from build123d import *

# Parameters (mm, degrees)
SKETCH1_R               = 7
BOSS_EXTRUDE1_DEPTH     = 13
SKETCH2_W               = 56.2
SKETCH2_H               = 16
CUT_EXTRUDE1_DEPTH      = 10
CUT_EXTRUDE2_REACH      = 56.246
SKETCH3_W               = 15
SKETCH3_H               = 16
SKETCH4_W               = 15
SKETCH4_H               = 23
BOSS_EXTRUDE2_DEPTH     = 16
SKETCH5_W               = 13
SKETCH5_H               = 21
CUT_EXTRUDE3_DEPTH      = 12
CUT_EXTRUDE4_REACH      = 59.303
SKETCH6_R               = 1.5
SKETCH6_R_2             = 1.05
SKETCH7_R               = 2.5
SKETCH7_R_2             = 1.5
BOSS_EXTRUDE3_DEPTH     = 10
CHAMFER1_SIZE           = 7
CHAMFER1_SIZE2          = 0.612420645
CUT_EXTRUDE5_REACH      = 103.55
CUT_EXTRUDE5_END_RADIUS = 7
SKETCH8_R               = 1.25
CUT_EXTRUDE6_REACH      = 103.55
CUT_EXTRUDE6_END_RADIUS = 7
SKETCH9_R               = 1.25


with BuildPart() as part:
    # Sketch1 → Boss-Extrude1 (new body)
    with BuildSketch(Plane(origin=(0, 0, 0), x_dir=(1, 0, 0), z_dir=(0, 1, 0))):
        Polygon((-28.1, -7), (-28.1, 10), (-48.1, 10), (-48.1, -23), (-28.1, -23), (28.1, -23), (48.1, -23), (48.1, 10), (28.1, 10), (28.1, -7), align=None)
        with Locations(Location((-38.1, 0, 0), (0, 0, 90))):
            Circle(SKETCH1_R, mode=Mode.SUBTRACT)
        with Locations(Location((38.1, 0, 0), (0, 0, 90))):
            Circle(SKETCH1_R, mode=Mode.SUBTRACT)
    extrude(amount=BOSS_EXTRUDE1_DEPTH)

    # Sketch2 → Cut-Extrude1 (cut)
    with BuildSketch(Plane(origin=(0, 13, 0), x_dir=(1, 0, 0), z_dir=(0, 1, 0))):
        with Locations((0, -15)):
            Rectangle(SKETCH2_W, SKETCH2_H)
    extrude(amount=-CUT_EXTRUDE1_DEPTH, mode=Mode.SUBTRACT)

    # Sketch3 → Cut-Extrude2 (cut, up to next)
    with BuildSketch(Plane(origin=(0, 3, 0), x_dir=(1, 0, 0), z_dir=(0, 1, 0)), mode=Mode.PRIVATE) as cut_extrude2_sk1:
        with Locations((0, -15)):
            Rectangle(SKETCH3_W, SKETCH3_H)
    cut_extrude2_tool1 = extrude(cut_extrude2_sk1.sketch, amount=-CUT_EXTRUDE2_REACH, mode=Mode.PRIVATE) & part.part
    add(cut_extrude2_tool1.solids().sort_by_distance((0, 3, 15))[0], mode=Mode.SUBTRACT)


with BuildPart() as cut_extrude2_piece_1:
    # of the separate pieces the step leaves, piece 1, a body of its own (cut_extrude2_pieces)
    add(part.part.solids().sort_by_distance((28.1, 0, 7))[0])



with BuildPart() as cut_extrude2_piece_2:
    # of the separate pieces the step leaves, piece 2, a body of its own (cut_extrude2_pieces)
    add(part.part.solids().sort_by_distance((-28.1, 0, 7))[0])


with BuildPart() as cut_extrude2_piece_1_1:
    add(cut_extrude2_piece_1.part)

    add(cut_extrude2_piece_2.part)  # Boss-Extrude2 merges Cut-Extrude2 piece 2
    # Sketch4 → Boss-Extrude2 (add)
    with BuildSketch(Plane.XY.offset(23)):
        with Locations((0, 11.5)):
            Rectangle(SKETCH4_W, SKETCH4_H)
    extrude(amount=-BOSS_EXTRUDE2_DEPTH)

    # Sketch5 → Cut-Extrude3 (cut)
    with BuildSketch(Plane.XY.offset(23)):
        with Locations((0, 11.5)):
            Rectangle(SKETCH5_W, SKETCH5_H)
    extrude(amount=-CUT_EXTRUDE3_DEPTH, mode=Mode.SUBTRACT)

    # Sketch6 → Cut-Extrude4 (cut, up to next)
    with BuildSketch(Plane.XY.offset(11), mode=Mode.PRIVATE) as cut_extrude4_sk1:
        with Locations((0, 11.464154045)):
            Circle(SKETCH6_R)
    cut_extrude4_tool1 = extrude(cut_extrude4_sk1.sketch, amount=-CUT_EXTRUDE4_REACH, mode=Mode.PRIVATE) & cut_extrude2_piece_1_1.part
    # Sketch6 → Cut-Extrude4 (cut, up to next)
    with BuildSketch(Plane.XY.offset(11), mode=Mode.PRIVATE) as cut_extrude4_sk2:
        with Locations((0, 6.964154045)):
            Circle(SKETCH6_R_2)
    cut_extrude4_tool2 = extrude(cut_extrude4_sk2.sketch, amount=-CUT_EXTRUDE4_REACH, mode=Mode.PRIVATE) & cut_extrude2_piece_1_1.part
    add(cut_extrude4_tool1.solids().sort_by_distance((0, 11.464154, 11))[0], mode=Mode.SUBTRACT)
    add(cut_extrude4_tool2.solids().sort_by_distance((0, 6.964154, 11))[0], mode=Mode.SUBTRACT)

    # Sketch7 → Boss-Extrude3 (add)
    with BuildSketch(Plane(origin=(0, 0, 7), x_dir=(-1, 0, 0), z_dir=(0, 0, -1))):
        with Locations(Location((0, 11.464154045, 0), (0, 0, 180))):
            Circle(SKETCH7_R)
        with Locations(Location((0, 11.464154045, 0), (0, 0, 180))):
            Circle(SKETCH7_R_2, mode=Mode.SUBTRACT)
    extrude(amount=BOSS_EXTRUDE3_DEPTH)

    # Chamfer1
    chamfer1_edges = [cut_extrude2_piece_1_1.edges().sort_by_distance(p)[0] for p in [
        (-2.5, 11.464154045, -3),
    ]]
    chamfer1_side = [cut_extrude2_piece_1_1.faces().sort_by_distance(p)[0] for p in [
        (-2.5, 11.464154045, 2),
    ]]
    chamfer(chamfer1_edges, length=CHAMFER1_SIZE, length2=CHAMFER1_SIZE2, reference=chamfer1_side[0])

    # Cut-Extrude5: up to this cylinder (the profile starts outside it)
    cut_extrude5_end = Plane(origin=(-38.1, 6.5, 0), z_dir=(0, -1, 0)) * Cylinder(CUT_EXTRUDE5_END_RADIUS, 222.1, mode=Mode.PRIVATE)
    # Sketch8 → Cut-Extrude5 (cut, up to the surface)
    with BuildSketch(Plane.ZY.offset(48.1), mode=Mode.PRIVATE) as cut_extrude5_sk1:
        with Locations((0, 6.5)):
            Circle(SKETCH8_R)
    cut_extrude5_tool1 = extrude(cut_extrude5_sk1.sketch, amount=-CUT_EXTRUDE5_REACH, mode=Mode.PRIVATE) - cut_extrude5_end
    add(cut_extrude5_tool1.solids().sort_by_distance((-48.1, 6.5, 0))[0], mode=Mode.SUBTRACT)

    # Cut-Extrude6: up to this cylinder (the profile starts outside it)
    cut_extrude6_end = Plane(origin=(38.1, 6.5, 0), z_dir=(0, -1, 0)) * Cylinder(CUT_EXTRUDE6_END_RADIUS, 222.1, mode=Mode.PRIVATE)
    # Sketch9 → Cut-Extrude6 (cut, up to the surface)
    with BuildSketch(Plane(origin=(48.1, 0, 0), x_dir=(0, 0, -1), z_dir=(1, 0, 0)), mode=Mode.PRIVATE) as cut_extrude6_sk1:
        with Locations(Location((0, 6.5, 0), (0, 0, 180))):
            Circle(SKETCH9_R)
    cut_extrude6_tool1 = extrude(cut_extrude6_sk1.sketch, amount=-CUT_EXTRUDE6_REACH, mode=Mode.PRIVATE) - cut_extrude6_end
    add(cut_extrude6_tool1.solids().sort_by_distance((48.1, 6.5, 0))[0], mode=Mode.SUBTRACT)


solid = cut_extrude2_piece_1_1.part
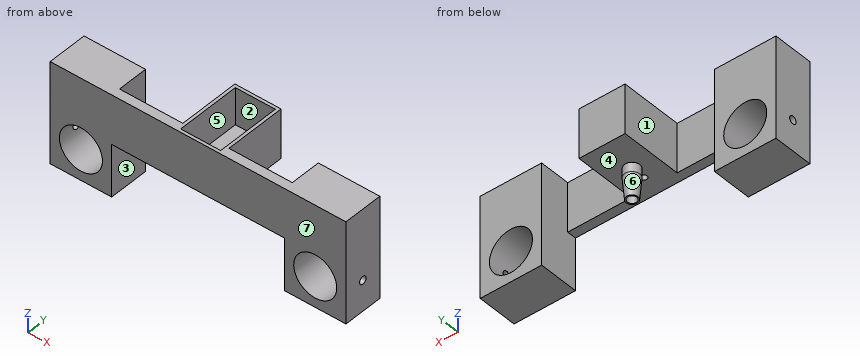
Input: part model. Units: mm. Frame: model coordinates. Face numbers are marked on the shaded views. A direction names the side the tool comes from. Give positions to 0.01 mm unless a question says otherwise; leave off trailing zeros. Write each loop counter-clockwise with the first axis right and the second up, starting at its lowest first coordinate (ties: lowest second). Pieces come first, ordered by that corner, then holes. Notation, with made-up numbers: M 0,17.5 L 15,17.5 A20 cw 15,49.5 Z; hole C 54.25,35.5 d7. An arc over 180 degrees is marked long. Write item = value, one per line. Start each with the question number.
1) Draft query along Y for the marked faces 4, 5, 6 and 7. Return one class per face: +Y half, -Y half, draft (parallel to the pull), parting line (faces both ways), or undercut.
2) Reachability of the marked faces 1, 2 and 3 from +Z, -Z, +X, -X, +Y, -Y: full face, straight path, thin tool, end or side. Return the list, or none.
3) Cut plane A-A on y = 4.25. Return the cut outline in (x, z).
4) Cut plane C-C on x = 0. Return the cut outline in (y, z), then the cut area to 3 significant figures.
5) Cut plane D-D on z = -5. Return the cut outline in (x, y), then the cut area to 3 significant figures.
6) First-contact query: pin 1 Ø3 at (y, z) = (6.5, 0) entering from -X; pin 2 Ø3.5 at (x, y) = (0, 6.96) entering from +Z; pin 3 Ø8 at (y, z) = (18.5, 7.5) entering from +X; pin 4 Ø5 at (x, z) = (17, 13) entering from +Y. Flat tips, straight axial feed; report the tip coordinate or a pass-through.
7) Material intervals for line 1 along X through (y, z) = (6.75, 19.5); line 2 along Y through (x, z) = (0, 8); line 3 along Z through (x, y) = (-38.1, 6.75), sorted ascending. Write a range as [from, to].
8) Cut plane B-B on z = 0. Return the cut outline in (x, y).
Solved:
q1.face_4 = draft
q1.face_5 = undercut
q1.face_6 = parting line
q1.face_7 = -Y half
q2.face_1 = +Z, -Z, +Y
q2.face_2 = +Z
q2.face_3 = -Z, +Y
q3.outline = M -48.1,-10 L -28.1,-10 L -28.1,23 L -48.1,23 Z; M -7.5,7 L 7.5,7 L 7.5,23 L 6.5,23 L 6.5,11 L -6.5,11 L -6.5,23 L -7.5,23 Z; M 28.1,-10 L 48.1,-10 L 48.1,23 L 28.1,23 Z; hole C -38.1,0 d14; hole C 38.1,0 d14
q4.outline = M 0,7 L 5.91,7 L 5.91,11 L 1,11 L 1,23 L 0,23 Z; M 8.01,7 L 8.96,7 L 8.96,4 L 9.58,-3 L 9.96,-3 L 9.96,11 L 8.01,11 Z; M 12.96,-3 L 13.35,-3 L 13.96,4 L 13.96,7 L 23,7 L 23,23 L 22,23 L 22,11 L 12.96,11 Z
q4.area = 111 mm2
q5.outline = M -48.1,0 L -43,0 L -43,13 L -48.1,13 Z; M -33.2,0 L -28.1,0 L -28.1,13 L -33.2,13 Z; M 28.1,0 L 33.2,0 L 33.2,13 L 28.1,13 Z; M 43,0 L 48.1,0 L 48.1,13 L 43,13 Z
q5.area = 265 mm2
q6.pin_1 = -48.1
q6.pin_2 = 11
q6.pin_3 = 7.5
q6.pin_4 = 3
q7.line_1 = [-48.1, -28.1], [-7.5, -6.5], [6.5, 7.5], [28.1, 48.1]
q7.line_2 = [0, 5.91], [8.01, 9.96], [12.96, 23]
q7.line_3 = [-10, -7], [7, 23]
q8.outline = M -48.1,0 L -45.1,0 L -45.1,5.25 L -48.1,5.25 Z; M -48.1,7.75 L -45.1,7.75 L -45.1,13 L -48.1,13 Z; M -31.1,0 L -28.1,0 L -28.1,13 L -31.1,13 Z; C 0,11.46 d4.3; M 28.1,0 L 31.1,0 L 31.1,13 L 28.1,13 Z; M 45.1,0 L 48.1,0 L 48.1,5.25 L 45.1,5.25 Z; M 45.1,7.75 L 48.1,7.75 L 48.1,13 L 45.1,13 Z; hole C 0,11.46 d3
